CAD build for the part. Positions are in the model's coordinates, mm. A direction names the side the tool comes from. Give positions to 0.01 mm unless a question says otherwise; leave off trailing zeros. Write each loop counter-clockwise with the first axis right and the second up, starting at its lowest first coordinate (ties: lowest second). Pieces come first, ordered by that corner, then holes. Notation, with made-up numbers: (88, 31) -> (143, 31) arc R12 ccw to (143, 54) -> close; hole circle Ø9 at (62.25, 61.25). An arc over 180 degrees is marked (long way). Answer as a JSON object with one key per item and string values.
```python
from build123d import *

# Parameters (mm, degrees)
BOSS_EXTRUDE1_DEPTH = 4
SKETCH2_W           = 12.35
SKETCH2_H           = 22.75
SKETCH2_W_2         = 12.2
SKETCH2_H_2         = 22.6
CUT_EXTRUDE10_DEPTH = 56.09122169
SKETCH6_R           = 4.5665
BOSS_EXTRUDE3_DEPTH = 10
SKETCH4_R           = 2.05
CUT_EXTRUDE11_DEPTH = 9.65
SKETCH15_R          = 1.3
CUT_EXTRUDE13_DEPTH = 9.65
SKETCH20_W          = 17.24
SKETCH20_H          = 7
BOSS_EXTRUDE4_DEPTH = 29.1
SKETCH14_R          = 2.05
CUT_EXTRUDE16_DEPTH = 58.586980363
SKETCH17_R          = 1.55
CUT_EXTRUDE17_DEPTH = 57.701346609


with BuildPart() as part:
    # Sketch1 → Boss-Extrude1 (new body)
    with BuildSketch(Plane.XY):
        Polygon((-16.687663097, 29.51713681), (16.687663097, 29.51713681), (29.751665716, 25.127138307), (45.48566771, 15.533136266), (46.115666453, 11.829137748), (44.06566621, 7.52513699), (39.527662855, 7.785135244), (26.057661336, 11.143136948), (19.095663738, 12.099134391), (13.943658967, -9.798863607), (14.617658977, -19.488863352), (14.549662185, -29.872864189), (-14.549662185, -29.872864189), (-14.619662252, -19.488863352), (-13.945660379, -9.798863607), (-19.097663288, 12.099134391), (-26.059662749, 11.143136948), (-39.529662405, 7.785135244), (-44.067662035, 7.52513699), (-46.113662247, 11.829137748), (-45.485663985, 15.533136266), (-29.75166199, 25.127138307), align=None)
    extrude(amount=BOSS_EXTRUDE1_DEPTH)

    # Sketch2 → Cut-Extrude10 (cut, through all)
    with BuildSketch(Plane.XY.offset(4)):
        with Locations((0.075, 1.67213681)):
            Rectangle(SKETCH2_W, SKETCH2_H)
        with Locations((0, 1.74713681)):
            Rectangle(SKETCH2_W_2, SKETCH2_H_2)
    extrude(amount=-CUT_EXTRUDE10_DEPTH, mode=Mode.SUBTRACT)

    # Sketch6 → Boss-Extrude3 (add)
    with BuildSketch(Plane.XY.offset(4)):
        with Locations((-41.008819859, 12.415108178)):
            Circle(SKETCH6_R)
        with Locations(Location((41.008819859, 12.415108178, 0), (0, 0, 180))):
            Circle(SKETCH6_R)
    extrude(amount=BOSS_EXTRUDE3_DEPTH)

    # Sketch4 → Cut-Extrude11 (cut)
    with BuildSketch(Plane.XY.offset(4)):
        with Locations((10.005, -26.272864189)):
            Circle(SKETCH4_R)
        with Locations((-10.005, -26.272864189)):
            Circle(SKETCH4_R)
    extrude(amount=-CUT_EXTRUDE11_DEPTH, mode=Mode.SUBTRACT)

    # Sketch15 → Cut-Extrude13 (cut)
    with BuildSketch(Plane.XY.offset(4)):
        with Locations((-0.026341033, -12.13286319)):
            Circle(SKETCH15_R)
        with Locations((-0.024336262, 15.52713681)):
            Circle(SKETCH15_R)
    extrude(amount=-CUT_EXTRUDE13_DEPTH, mode=Mode.SUBTRACT)

    # Sketch20 → Boss-Extrude4 (add)
    with BuildSketch(Plane(origin=(14.744644235, -0.096551274, 0), x_dir=(0, 0, -1), z_dir=(0.9999785610524021, -0.006548086405005186, 0))):
        with Locations((-12.62, -26.276951301)):
            Rectangle(SKETCH20_W, SKETCH20_H)
    extrude(amount=-BOSS_EXTRUDE4_DEPTH)

    # Sketch14 → Cut-Extrude16 (cut, through all)
    with BuildSketch(Plane.XY.offset(4)):
        with Locations((-10.005, -26.272864189)):
            Circle(SKETCH14_R)
        with Locations((10.005, -26.272864189)):
            Circle(SKETCH14_R)
    extrude(amount=CUT_EXTRUDE16_DEPTH, mode=Mode.SUBTRACT)

    # Sketch17 → Cut-Extrude17 (cut, through all)
    with BuildSketch(Plane.XY.offset(14)):
        with Locations((41.008819859, 12.415108178)):
            Circle(SKETCH17_R)
        with Locations(Location((-41.008819859, 12.415108178, 0), (0, 0, 180))):
            Circle(SKETCH17_R)
    extrude(amount=-CUT_EXTRUDE17_DEPTH, mode=Mode.SUBTRACT)


solid = part.part
```
1) 3-axis set-ups, long thin cutter, end or side, ignore diameter. For faces 1 (the flat face through (-14.287, -14.712, 1.972)), 2 (the flat face through (14.276, -14.576, 1.972)), 3 (the flat face through (32.89, 9.44, 1.97)), 4 (the flat face through (6.25, 2, 2)), 5 (the cylindrical face through (45.57, 12.21, 8.93)): which of +Z, -Z, +X, -X, +Y, -Y reach the whole face in a straight line?
Model answer:
{"face 1": "+Z, -Z, -X", "face 2": "+Z, -Z, +X", "face 3": "+Z, -Z, -Y", "face 4": "+Z, -Z", "face 5": "+Z"}
2) Slice it at A-A (z = 7.25). State how many separate pieces and enclosed holes the cut face has, then the cut area to 3 significant figures.
Model answer:
{"separate pieces": "3", "enclosed holes": "4", "area": "293 mm2"}
3) Pin check, flat tips, straight feed: pin 1 (6 mm diameter, centred on x = -12.5, y = -1, fed in from +Z); pin 2 (2.5 mm diameter, centred on x = 10.01, y = -26.27, fed in from -Z); pin 3 (1.5 mm diameter, centred on x = -35, z = 3, fed in from -Y); pin 4 (8 mm diameter, centred on y = 1.5, z = 5.5, fed in from -X). Stop position of each tip, or through.
Model answer:
{"pin 1": "stops at z = 4", "pin 2": "passes through", "pin 3": "stops at y = 8.73", "pin 4": "stops at x = -17.48"}
4) Slice it at D-D (y = -4). List the corners of the cut face in (x, z), then the cut area to 3 significant figures.
Model answer:
{"outline": "(-15.31, 0) -> (-6.1, 0) -> (-6.1, 4) -> (-15.31, 4) -> close; (6.25, 0) -> (15.31, 0) -> (15.31, 4) -> (6.25, 4) -> close", "area": "73.1 mm2"}
5) Slice it at C-C (y = 9.5). List the corners of the cut face in (x, z).
Model answer:
{"outline": "(-45.01, 0) -> (-32.65, 0) -> (-32.65, 4) -> (-37.49, 4) -> (-37.49, 14) -> (-44.52, 14) -> (-44.52, 4) -> (-45.01, 4) -> close; (-18.49, 0) -> (-6.1, 0) -> (-6.1, 4) -> (-18.49, 4) -> close; (6.25, 0) -> (18.48, 0) -> (18.48, 4) -> (6.25, 4) -> close; (32.65, 0) -> (45.01, 0) -> (45.01, 4) -> (44.52, 4) -> (44.52, 14) -> (37.49, 14) -> (37.49, 4) -> (32.65, 4) -> close"}
6) Slice it at B-B (x = 5). List the corners of the cut face in (y, z), then the cut area to 3 significant figures.
Model answer:
{"outline": "(-29.87, 0) -> (-9.7, 0) -> (-9.7, 4) -> (-22.81, 4) -> (-22.81, 21.24) -> (-29.81, 21.24) -> (-29.81, 4) -> (-29.87, 4) -> close; (13.05, 0) -> (29.52, 0) -> (29.52, 4) -> (13.05, 4) -> close", "area": "267 mm2"}
7) Wall check: probe 1 along Z at (x, y) = (11, 0); probe 2 along Y at (x, z) = (10.5, 17.75); probe 3 along X at (y, z) = (-20, 1.5). Give the ranges that are in metal, low to high.
Model answer:
{"probe 1": "z = 0 to 4", "probe 2": "y = -29.85 to -28.26, -24.28 to -22.85", "probe 3": "x = -14.62 to 14.61"}
8) Mould opens along X. For faces 6 (the cylindrical face through (-45.57, 12.62, 8.93)), 7 (the flat face through (0, -26, 21.24)), 8 (the flat face through (37.509, 20.397, 1.972)) say: released by +X, released by -X, zero draft, split by the parting line, or undercut.
Model answer:
{"face 6": "undercut", "face 7": "zero draft", "face 8": "released by +X"}
